Source: CAD feature listing. Evaluate the final solid. Frame: model axes, mm. A direction names the side the tool comes from. Give positions to 0.01 mm unless a question says otherwise; leave off trailing zeros. Write each loop counter-clockwise with the first axis right and the second up, starting at its lowest first coordinate (ties: lowest second). Pieces come first, ordered by that corner, then holes.
```python
from build123d import *

# Parameters (mm, degrees)
F0_W     = 279.4
F0_H     = 25.4
F1_DEPTH = 25.4
F3_DEPTH = 279.4
F4_R     = 6.35
F5_DEPTH = 25.4
F6_W     = 5.08
F6_H     = 20.8788
F6_W_2   = 46.6979
F6_H_2   = 5.08
F7_DEPTH = 2.54


with BuildPart() as f1:
    # F0 (on Front) → F1 (new body)
    with BuildSketch(Plane.XZ):
        with Locations((139.7, 12.7)):
            Rectangle(F0_W, F0_H)
    extrude(amount=-F1_DEPTH)

    # F2 (on face) → F3 (cut)
    with BuildSketch(Plane(origin=(0, 0, 0), x_dir=(0, -1, 0), z_dir=(-1, 0, 0))):
        with BuildLine():
            Line((0, 0), (0, 12.7))
            ThreePointArc((0, 12.7), (-3.719744, 3.719744), (-12.7, 0))
            Line((-12.7, 0), (0, 0))
        make_face()
        with BuildLine():
            Line((-25.4, 0), (-12.7, 0))
            ThreePointArc((-12.7, 0), (-21.680256, 3.719744), (-25.4, 12.7))
            Line((-25.4, 12.7), (-25.4, 0))
        make_face()
        with BuildLine():
            ThreePointArc((-25.4, 12.7), (-21.680256, 21.680256), (-12.7, 25.4))
            Line((-12.7, 25.4), (-25.4, 25.4))
            Line((-25.4, 25.4), (-25.4, 12.7))
        make_face()
        with BuildLine():
            ThreePointArc((-12.7, 25.4), (-3.719744, 21.680256), (0, 12.7))
            Line((0, 12.7), (0, 25.4))
            Line((0, 25.4), (-12.7, 25.4))
        make_face()
    extrude(amount=-F3_DEPTH, mode=Mode.SUBTRACT)

    # F4 (on Right) → F5 (cut)
    with BuildSketch(Plane.YZ):
        with Locations((12.7, 12.7)):
            Circle(F4_R)
    extrude(amount=F5_DEPTH, mode=Mode.SUBTRACT)

    # F6 (on face) → F7 (cut)
    with BuildSketch(Plane(origin=(0, 0, 0), x_dir=(0, -1, 0), z_dir=(-1, 0, 0))):
        with Locations((-12.623682, 25.426102)):
            Rectangle(F6_W, F6_H)
        with Locations((13.265268, 12.446702)):
            Rectangle(F6_W_2, F6_H_2)
        with Locations((-38.512632, 12.446702)):
            Rectangle(F6_W_2, F6_H_2)
        with Locations((-12.623682, -0.532698)):
            Rectangle(F6_W, F6_H)
    extrude(amount=-F7_DEPTH, mode=Mode.SUBTRACT)


solid = f1.part
```
1. Pin query (flat end, axial travel): P1, Ø2.5, axis at y = 23.5, z = 13.5, coming from the -X side; P2, Ø3, axis at x = 1, y = 3.5, coming from the +Z side; P3, Ø2, axis at x = 0.5, z = 4.5, coming from the -Y side. Return the tip coordinate at first contact, or that it passes through.
2. Section query A-A (z = 4). Return loops of the section in (x, y).
3. Pull-direction query (Z, two-part tool) for faces 1 (the cylindrical face through (12.522, 6.356, 12.979)), 2 (the flat face through (279.4, 13, 13)); classes: pulls with the +Z half, pulls with the -Z half, needs draft (parallel to the pull), parting line crosses it, or undercut.
4. Access query for faces 3 (the flat face through (25.4, 13, 13)), 4 (the flat face through (2.54, 4, 12)), 5 (the flat face through (2.54, 13, 4)), 6 (the flat face through (0, 19, 6)). Directions: +Z, -Z, +X, -X, +Y, -Y. A direction counts if a zero-diameter tool reaches every point of the face in a straight line with its end or side. Return the directions, or none.
5. Section query B-B (x = 178.5). Return loops of the section in (y, z), plus the area to 3 significant figures.
6. Section query C-C (y = 4). Return loops of the section in (x, z), plus the area to 3 significant figures.
7. Line query: probe 1 along Z at (x, y) = (11.75, 12.7); probe 2 along X at (y, z) = (11.25, 2.25). Output: solid intervals per line, ascending.
The answers:
1. P1: stops at x = 2.54
1. P2: stops at z = 22.8
1. P3: stops at y = 2.24
2. outline: (0, 3.45) - (279.4, 3.45) - (279.4, 21.95) - (0, 21.95) - (0, 15.16) - (2.54, 15.16) - (2.54, 10.08) - (0, 10.08) - close
3. face 1: undercut
3. face 2: needs draft
4. face 3: -X
4. face 4: -X, +Y, -Y
4. face 5: +Z, -Z, -X
4. face 6: +Z, -Z, -X, +Y, -Y
5. outline: circle Ø25.4 at (12.7, 12.7)
5. area: 507 mm2
6. outline: (0, 3.45) - (279.4, 3.45) - (279.4, 21.95) - (0, 21.95) - (0, 14.99) - (2.54, 14.99) - (2.54, 9.91) - (0, 9.91) - close
6. area: 5,160 mm2
7. probe 1: z = 0 to 6.35, 19.05 to 25.4
7. probe 2: x = 2.54 to 279.4
